Geometry: final body of the model. Coordinates: model frame, mm. A direction names the side the tool comes from. Coordinates: 2 decimals unless noted, no trailing zeros. Loops run counter-clockwise (first coordinate to the right, second up) from the corner with the lowest first, then second, coordinate; pieces in that order, holes last. Notation, with made-up numbers: (30, -26) -> (85, -26) arc R18 ccw to (85, -12) -> close; hole circle Ø8 at (34.5, 83). An arc over 180 degrees is marked (long way). One line per item, written item: value. Start each with the question number.
Item 1: Section query C-C on z = -1. Return loops of the section in (x, y), then the cut area to 3 significant figures.
Item 2: Set-up query: faces 1 (the flat face through (3.23, 2.8, -3.55)), 2 (the flat face through (4.1, 3, -3.5)), 3 (the flat face through (4, 0.8, -3)). Return all of +Z, -Z, +X, -X, +Y, -Y with unobstructed straight access to the full face (end or side cutting, diameter ignored); none if empty.
Item 3: Section query A-A on y = 2.7. Return loops of the section in (x, z).
Item 4: Section query B-B on x = 1.25. Return loops of the section in (y, z), then the cut area to 3 significant figures.
Item 5: Ray query, probe 1 along X at (y, z) = (0.45, -3.5) (3 decimals); probe 2 along X at (y, z) = (0.2, -3.5); probe 3 along Z at (x, y) = (4, 0.6). Return the intervals inside material, ascending. Write a range as from..to.
Item 6: Mould query, pull axis X, two halves, no side actions, for faces 4 (the flat face through (3.75, 2.8, -3.6)), 5 (the cylindrical face through (4.041, 0.394, -5.217)), 6 (the flat face through (6.655, 1.479, -3.451)), 7 (the flat face through (3.451, 1.479, -0.345)). Classes: +X half, -X half, draft (parallel to the pull), parting line (faces both ways), or undercut.
Item 7: Contact query for a flat-ended pin moving along its axis: pin 1 Ø3 at (x, z) = (3.5, -3.5) entering from -Y. Output: stop coordinate, or through.
Item 8: Section query D-D on y = 0.3. Return loops of the section in (x, z).
from build123d import *

# Parameters (mm, degrees)
SKETCH1_W           = 7
SKETCH1_H           = 7
BOSS_EXTRUDE1_DEPTH = 3
CUT_EXTRUDE1_DEPTH  = 7
CUT_EXTRUDE2_DEPTH  = 11
SKETCH4_R           = 1.8
CUT_EXTRUDE3_DEPTH  = 0.8
CUT_EXTRUDE4_DEPTH  = 0.4


with BuildPart() as part:
    # Sketch1 → Boss-Extrude1 (new body)
    with BuildSketch(Plane(origin=(0, 0, 0), x_dir=(1, 0, 0), z_dir=(0, 1, 0))):
        with Locations((3.5, 3.5)):
            Rectangle(SKETCH1_W, SKETCH1_H)
    extrude(amount=BOSS_EXTRUDE1_DEPTH)

    # Sketch2 → Cut-Extrude1 (cut)
    with BuildSketch(Plane.XY):
        Polygon((0, 0), (0.7, 3), (0, 3), align=None)
        Polygon((7, 0), (6.3, 3), (7, 3), align=None)
    extrude(amount=-CUT_EXTRUDE1_DEPTH, mode=Mode.SUBTRACT)

    # Sketch3 → Cut-Extrude2 (cut)
    with BuildSketch(Plane(origin=(0, 0, 0), x_dir=(0, 0, -1), z_dir=(1, 0, 0))):
        Polygon((0, 0), (0.7, 3), (0, 3), align=None)
        Polygon((7, 3), (6.3, 3), (7, 0), align=None)
    extrude(amount=CUT_EXTRUDE2_DEPTH, mode=Mode.SUBTRACT)

    # Sketch4 → Cut-Extrude3 (cut)
    with BuildSketch(Plane.XZ):
        with Locations(Location((3.5, -3.5, 0), (0, 0, 270))):
            Circle(SKETCH4_R)
    extrude(amount=-CUT_EXTRUDE3_DEPTH, mode=Mode.SUBTRACT)

    # Sketch6 → Cut-Extrude4 (cut)
    with BuildSketch(Plane(origin=(0, 3, 0), x_dir=(1, 0, 0), z_dir=(0, 1, 0))):
        Polygon((2.811280801, 1.826752028), (3.664546025, 5.326752028), (4.171457083, 5.326752028), (3.318892981, 1.826752028), align=None)
    extrude(amount=-CUT_EXTRUDE4_DEPTH, mode=Mode.SUBTRACT)


solid = part.part
Reply:
1. outline: (0, 0) -> (7, 0) -> (6.3, 3) -> (0.7, 3) -> close
1. area: 18.9 mm²
2. face 1: +Y
2. face 2: +Z, -Z, +X, -X, +Y
2. face 3: -Y
3. outline: (0.63, -6.37) -> (6.37, -6.37) -> (6.37, -0.63) -> (0.63, -0.63) -> close; hole (2.81, -1.83) -> (3.66, -5.33) -> (4.17, -5.33) -> (3.32, -1.83) -> close
4. outline: (0, -7) -> (3, -6.3) -> (3, -0.7) -> (0, 0) -> close
4. area: 18.9 mm²
5. probe 1: x = 0.105..1.7, 5.3..6.895
5. probe 2: x = 0.05..1.7, 5.3..6.95
5. probe 3: z = -6.86..-5.23, -1.77..-0.14
6. face 4: undercut
6. face 5: undercut
6. face 6: +X half
6. face 7: draft
7. pin 1: stops at y = 0.8
8. outline: (0.07, -6.93) -> (6.93, -6.93) -> (6.93, -0.07) -> (0.07, -0.07) -> close; hole circle Ø3.6 at (3.5, -3.5)
